Here's the drawing with two shaded views (mm, measured from the low corner). I have some questions. Coordinates: 2 decimals unless noted, no trailing zeros. Write each loop counter-clockwise with the first axis right and the second up, starting at its lowest first coordinate (ties: lowest second). Pieces come first, ordered by that corner, then holes.
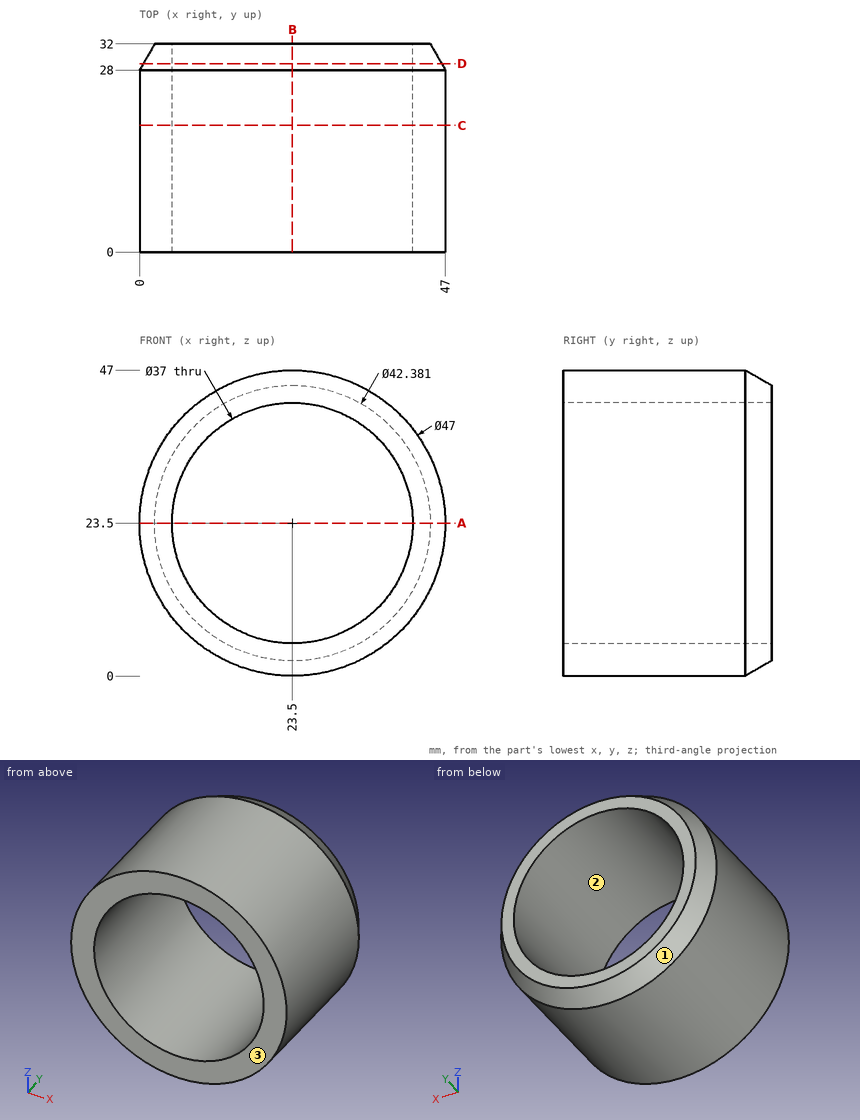
1. I'm going to push flat-ended pins straight in: P1, Ø3, axis at x = 31.5, y = 23.5, coming from the -Z side; P2, Ø6, axis at x = 33.5, y = 25.5, coming from the -Z side; P3, Ø1.5, axis at x = 22.5, y = 7.5, coming from the +Z side. Where does each tip first touch, or does it pass through?
2. If we section it at D-D, the plane y = 29: List the corners of the cut face in (x, z) for me (1 decimal).
3. If we section it at C-C, the plane y = 19.5: List the corners of the cut face in (x, z) for me.
4. We'd pull the mould along Z, two halves only. Please class the marked faces 1, 2 and 3: released by +Z, released by -Z, zero draft, split by the parting line, or undercut.
5. If we section it at A-A, the plane z = 23.5: List the corners of the cut face in (x, y) for me, plus the area to 3 significant figures.
6. If we section it at B-B, the plane x = 23.5: List the corners of the cut face in (y, z) for me, plus the area to 3 significant figures.
7. If I drill on L1, parallel to X at y = 14, z = 23.5; L2, parallel to Z at x = 19.5, y = 12.5, over which ranges is the centre line in solid material (lowest first)?
Answers:
1. P1: stops at z = 0.92
1. P2: stops at z = 1.07
1. P3: stops at z = 47
2. outline: circle Ø45.8 at (23.5, 23.5); hole circle Ø37 at (23.5, 23.5)
3. outline: circle Ø47 at (23.5, 23.5); hole circle Ø37 at (23.5, 23.5)
4. face 1: split by the parting line
4. face 2: undercut
4. face 3: zero draft
5. outline: (0, 0) - (5, 0) - (5, 32) - (2.31, 32) - (0, 28) - close; (42, 0) - (47, 0) - (47, 28) - (44.69, 32) - (42, 32) - close
5. area: 311 mm2
6. outline: (0, 0) - (28, 0) - (32, 2.31) - (32, 5) - (0, 5) - close; (0, 42) - (32, 42) - (32, 44.69) - (28, 47) - (0, 47) - close
6. area: 311 mm2
7. L1: x = 0 to 5, 42 to 47
7. L2: z = 0.34 to 5.44, 41.56 to 46.66
